For this review, take the finished solid that the model builds, in its own axes (mm). Face numbers are marked on the shaded views. Coordinates: 2 decimals unless noted, no trailing zeros. Order: outer loops, then holes, each group sorted by start corner. A loop starts at its lowest first (then second) coordinate and runs counter-clockwise, first axis right, second up. Notation, with made-up numbers: M -24,-33 L 8,-33 A20 cw 8,-29 Z; hole C 86,-33.75 d10. An arc over 180 degrees is marked long. Use one line per item in the form item = value. Start each with the question number.
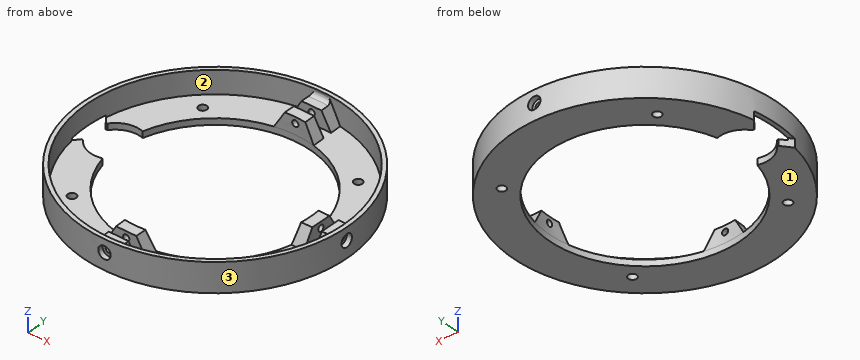
```python
from build123d import *
from OCP.BRepFilletAPI import BRepFilletAPI_MakeChamfer

# Parameters (mm, degrees)
CUT_EXTRUDE1_DEPTH             = 4
CHAMFER1_SIZE                  = 4.528404541
BOSS_EXTRUDE1_START            = 8
BOSS_EXTRUDE1_DEPTH            = 8
CHAMFER2_SIZE                  = 8
CHAMFER2_SIZE_2                = 4.618802154
CIRPATTERN1_COUNT              = 3
CIRPATTERN1_ANGLE              = 180
CHAMFER2_OF_CIRPATTERN1_SIZE   = 8
CHAMFER2_OF_CIRPATTERN1_SIZE_2 = 4.618802154
FILLET1_R                      = 2
SKETCH4_R                      = 2
CUT_EXTRUDE2_DEPTH             = 10
SKETCH5_R                      = 1.5
CUT_EXTRUDE3_DEPTH             = 158
SKETCH7_R                      = 3
CUT_EXTRUDE5_DEPTH             = 4
CIRPATTERN3_COUNT              = 3
CIRPATTERN3_ANGLE              = 180


# Some blends are built 0.0001 mm under size
with BuildPart() as part:
    # Sketch1 → Revolve1 (revolve)
    with BuildSketch(Plane(origin=(0, 0, 0), x_dir=(1, 0, 0), z_dir=(0, 1, 0))):
        Polygon((-46, 0), (-46, -3), (-61.5, -3), (-61.5, -14), (-63.5, -14), (-63.5, 0), align=None)
    revolve(axis=Axis((0, 0, 0.5), (0, 0, 1)))

    # Sketch2 → Cut-Extrude1 (cut)
    with BuildSketch(Plane(origin=(0, 0, 0), x_dir=(-1, 0, 0), z_dir=(0, 0, -1))):
        with BuildLine():
            Line((57.746794345, 7), (73.255615774, 7))
            Line((73.255615774, 7), (73.255615774, -7))
            Line((73.255615774, -7), (57.746794345, -7))
            ThreePointArc((57.746794345, -7), (36, 0), (57.746794345, 7))
        make_face()
    extrude(amount=-CUT_EXTRUDE1_DEPTH, mode=Mode.SUBTRACT)

    # Chamfer1
    # the kernel refuses this chamfer: 5, 4.528404541 mm, written as the material it takes off along each edge
    with BuildSketch(Plane(origin=(-63.112993908, -7, 4), x_dir=(1, 0, 0), z_dir=(0, 0, -1))) as chamfer1_piece_1:
        with BuildLine():
            Line((CHAMFER1_SIZE, 0), (0.712866483, 4.767501749))
            ThreePointArc((0.712866483, 4.767501749), (0.321261242, 2.457711608), (0, 0))
            Line((0, 0), (CHAMFER1_SIZE, 0))
        make_face()
    extrude(amount=16.39656237, mode=Mode.SUBTRACT)
    with BuildSketch(Plane(origin=(-63.112993908, 7, 4), x_dir=(1, 0, 0), z_dir=(0, 0, -1))) as chamfer1_piece_2:
        with BuildLine():
            Line((CHAMFER1_SIZE, 0), (0.712866483, -4.767501749))
            ThreePointArc((0.712866483, -4.767501749), (0.321261242, -2.457711608), (0, 0))
            Line((0, 0), (CHAMFER1_SIZE, 0))
        make_face()
    extrude(amount=16.39656237, mode=Mode.SUBTRACT)

    # Sketch3 → Boss-Extrude1 (add)
    with BuildSketch(Plane.XY.offset(3).offset(BOSS_EXTRUDE1_START)):
        with BuildLine():
            Line((-9.502273243, -50.959479433), (-9.711670224, -44.963134471))
            ThreePointArc((-9.711670224, -44.963134471), (-0.109415415, -45.999869872), (9.497662676, -45.008825842))
            Line((9.497662676, -45.008825842), (9.497662676, -51.008825842))
            Line((9.497662676, -51.008825842), (-9.502273243, -50.959479433))
        make_face()
        with BuildLine():
            Line((9.497662676, -55.408840682), (-9.348607402, -55.359893372))
            Line((-9.348607402, -55.359893372), (-9.158135478, -60.814295643))
            ThreePointArc((-9.158135478, -60.814295643), (0.171750649, -61.499760176), (9.497662676, -60.762195514))
            Line((9.497662676, -60.762195514), (9.497662676, -55.408840682))
        make_face()
    boss_extrude1 = extrude(amount=-BOSS_EXTRUDE1_DEPTH)

    # Chamfer2
    chamfer2_edges_1 = [part.edges().sort_by_distance(p)[0] for p in [
        (-9.25337144, -58.087094508, 11),
    ]]
    chamfer2_side_1 = [part.faces().sort_by_distance(p)[0] for p in [
        (-9.25337144, -58.087094508, 10.907623957),
    ]]
    chamfer2_edges_2 = [part.edges().sort_by_distance(p)[0] for p in [
        (-9.606971733, -47.961306952, 11),
    ]]
    chamfer2_side_2 = [part.faces().sort_by_distance(p)[0] for p in [
        (-9.606971733, -47.961306952, 10.907623957),
    ]]
    chamfer2_edges_3 = [part.edges().sort_by_distance(p)[0] for p in [
        (9.497662676, -48.008825842, 11),
    ]]
    chamfer2_side_3 = [part.faces().sort_by_distance(p)[0] for p in [
        (9.497662676, -48.008825842, 10.907623957),
    ]]
    chamfer2_edges_4 = [part.edges().sort_by_distance(p)[0] for p in [
        (9.497662676, -58.085518098, 11),
    ]]
    chamfer2_side_4 = [part.faces().sort_by_distance(p)[0] for p in [
        (9.497662676, -58.085518098, 10.907623957),
    ]]
    chamfer2 = BRepFilletAPI_MakeChamfer(part.part.solid().wrapped)
    for e in chamfer2_edges_1:
        chamfer2.Add(CHAMFER2_SIZE - 0.0001, CHAMFER2_SIZE_2 - 0.0001, e.wrapped, chamfer2_side_1[0].wrapped)
    for e in chamfer2_edges_2:
        chamfer2.Add(CHAMFER2_SIZE - 0.0001, CHAMFER2_SIZE_2 - 0.0001, e.wrapped, chamfer2_side_2[0].wrapped)
    for e in chamfer2_edges_3:
        chamfer2.Add(CHAMFER2_SIZE - 0.0001, CHAMFER2_SIZE_2 - 0.0001, e.wrapped, chamfer2_side_3[0].wrapped)
    for e in chamfer2_edges_4:
        chamfer2.Add(CHAMFER2_SIZE - 0.0001, CHAMFER2_SIZE_2 - 0.0001, e.wrapped, chamfer2_side_4[0].wrapped)
    add(Compound.cast(chamfer2.Shape()), mode=Mode.REPLACE)  # a hair under: the kernel refuses the full size

    # CirPattern1: Boss-Extrude1 ×3 about axis
    cirpattern1_axis = Axis((0, 0, 0), (0, 0, 1))
    for i in range(1, CIRPATTERN1_COUNT):
        add(boss_extrude1.rotate(cirpattern1_axis, i * CIRPATTERN1_ANGLE / (CIRPATTERN1_COUNT - 1)))

    # Chamfer2 of CirPattern1
    chamfer2_of_cirpattern1_edges_1 = [part.edges().sort_by_distance(p)[0] for p in [
        (58.087094508, -9.25337144, 11),
    ]]
    chamfer2_of_cirpattern1_side_1 = [part.faces().sort_by_distance(p)[0] for p in [
        (58.087094508, -9.25337144, 10.907623957),
    ]]
    chamfer2_of_cirpattern1_edges_2 = [part.edges().sort_by_distance(p)[0] for p in [
        (47.961306952, -9.606971733, 11),
    ]]
    chamfer2_of_cirpattern1_side_2 = [part.faces().sort_by_distance(p)[0] for p in [
        (47.958083075, -9.514651963, 11),
    ]]
    chamfer2_of_cirpattern1_edges_3 = [part.edges().sort_by_distance(p)[0] for p in [
        (48.008825842, 9.497662676, 11),
    ]]
    chamfer2_of_cirpattern1_side_3 = [part.faces().sort_by_distance(p)[0] for p in [
        (48.008825842, 9.497662676, 10.907623957),
    ]]
    chamfer2_of_cirpattern1_edges_4 = [part.edges().sort_by_distance(p)[0] for p in [
        (58.085518098, 9.497662676, 11),
    ]]
    chamfer2_of_cirpattern1_side_4 = [part.faces().sort_by_distance(p)[0] for p in [
        (58.085518098, 9.497662676, 10.907623957),
    ]]
    chamfer2_of_cirpattern1_edges_5 = [part.edges().sort_by_distance(p)[0] for p in [
        (9.25337144, 58.087094508, 11),
    ]]
    chamfer2_of_cirpattern1_side_5 = [part.faces().sort_by_distance(p)[0] for p in [
        (9.25337144, 58.087094508, 10.907623957),
    ]]
    chamfer2_of_cirpattern1_edges_6 = [part.edges().sort_by_distance(p)[0] for p in [
        (9.606971733, 47.961306952, 11),
    ]]
    chamfer2_of_cirpattern1_side_6 = [part.faces().sort_by_distance(p)[0] for p in [
        (9.606971733, 47.961306952, 10.907623957),
    ]]
    chamfer2_of_cirpattern1_edges_7 = [part.edges().sort_by_distance(p)[0] for p in [
        (-9.497662676, 48.008825842, 11),
    ]]
    chamfer2_of_cirpattern1_side_7 = [part.faces().sort_by_distance(p)[0] for p in [
        (-9.497662676, 48.008825842, 10.907623957),
    ]]
    chamfer2_of_cirpattern1_edges_8 = [part.edges().sort_by_distance(p)[0] for p in [
        (-9.497662676, 58.085518098, 11),
    ]]
    chamfer2_of_cirpattern1_side_8 = [part.faces().sort_by_distance(p)[0] for p in [
        (-9.497662676, 58.085518098, 10.907623957),
    ]]
    chamfer2_of_cirpattern1 = BRepFilletAPI_MakeChamfer(part.part.solid().wrapped)
    for e in chamfer2_of_cirpattern1_edges_1:
        chamfer2_of_cirpattern1.Add(CHAMFER2_OF_CIRPATTERN1_SIZE - 0.0001, CHAMFER2_OF_CIRPATTERN1_SIZE_2 - 0.0001, e.wrapped, chamfer2_of_cirpattern1_side_1[0].wrapped)
    for e in chamfer2_of_cirpattern1_edges_2:
        chamfer2_of_cirpattern1.Add(CHAMFER2_OF_CIRPATTERN1_SIZE_2 - 0.0001, CHAMFER2_OF_CIRPATTERN1_SIZE - 0.0001, e.wrapped, chamfer2_of_cirpattern1_side_2[0].wrapped)
    for e in chamfer2_of_cirpattern1_edges_3:
        chamfer2_of_cirpattern1.Add(CHAMFER2_OF_CIRPATTERN1_SIZE - 0.0001, CHAMFER2_OF_CIRPATTERN1_SIZE_2 - 0.0001, e.wrapped, chamfer2_of_cirpattern1_side_3[0].wrapped)
    for e in chamfer2_of_cirpattern1_edges_4:
        chamfer2_of_cirpattern1.Add(CHAMFER2_OF_CIRPATTERN1_SIZE - 0.0001, CHAMFER2_OF_CIRPATTERN1_SIZE_2 - 0.0001, e.wrapped, chamfer2_of_cirpattern1_side_4[0].wrapped)
    for e in chamfer2_of_cirpattern1_edges_5:
        chamfer2_of_cirpattern1.Add(CHAMFER2_OF_CIRPATTERN1_SIZE - 0.0001, CHAMFER2_OF_CIRPATTERN1_SIZE_2 - 0.0001, e.wrapped, chamfer2_of_cirpattern1_side_5[0].wrapped)
    for e in chamfer2_of_cirpattern1_edges_6:
        chamfer2_of_cirpattern1.Add(CHAMFER2_OF_CIRPATTERN1_SIZE - 0.0001, CHAMFER2_OF_CIRPATTERN1_SIZE_2 - 0.0001, e.wrapped, chamfer2_of_cirpattern1_side_6[0].wrapped)
    for e in chamfer2_of_cirpattern1_edges_7:
        chamfer2_of_cirpattern1.Add(CHAMFER2_OF_CIRPATTERN1_SIZE - 0.0001, CHAMFER2_OF_CIRPATTERN1_SIZE_2 - 0.0001, e.wrapped, chamfer2_of_cirpattern1_side_7[0].wrapped)
    for e in chamfer2_of_cirpattern1_edges_8:
        chamfer2_of_cirpattern1.Add(CHAMFER2_OF_CIRPATTERN1_SIZE - 0.0001, CHAMFER2_OF_CIRPATTERN1_SIZE_2 - 0.0001, e.wrapped, chamfer2_of_cirpattern1_side_8[0].wrapped)
    add(Compound.cast(chamfer2_of_cirpattern1.Shape()), mode=Mode.REPLACE)  # a hair under: the kernel refuses the full size

    # Fillet1
    fillet1_edges = [part.edges().sort_by_distance(p)[0] for p in [
        (0.180770138, -61.499734326, 11),
        (61.499734326, 0.180770138, 11),
        (-0.180770138, 61.499734326, 11),
    ]]
    fillet(fillet1_edges, radius=FILLET1_R)

    # Sketch4 → Cut-Extrude2 (cut)
    with BuildSketch(Plane(origin=(0, 0, 0), x_dir=(-1, 0, 0), z_dir=(0, 0, -1))):
        with Locations((-37.476659403, 37.476659403)):
            Circle(SKETCH4_R)
        with Locations((37.476659403, 37.476659403)):
            Circle(SKETCH4_R)
        with Locations((37.476659403, -37.476659403)):
            Circle(SKETCH4_R)
        with Locations((-37.476659403, -37.476659403)):
            Circle(SKETCH4_R)
    extrude(amount=-CUT_EXTRUDE2_DEPTH, mode=Mode.SUBTRACT)

    # Sketch5 → Cut-Extrude3 (cut)
    with BuildSketch(Plane(origin=(0, 0, 0), x_dir=(1, 0, 0), z_dir=(0, 1, 0))):
        with Locations(Location((0, -8, 0), (0, 0, 270))):
            Circle(SKETCH5_R)
    cut_extrude3 = extrude(amount=-CUT_EXTRUDE3_DEPTH, mode=Mode.SUBTRACT)

    # Sketch7 → Cut-Extrude5 (cut)
    with BuildSketch(Plane(origin=(0, -65, 0), x_dir=(1, 0, 0), z_dir=(0, 1, 0))):
        with Locations(Location((0, -8, 0), (0, 0, 90))):
            Circle(SKETCH7_R)
    cut_extrude5 = extrude(amount=CUT_EXTRUDE5_DEPTH, mode=Mode.SUBTRACT)

    # CirPattern3: Cut-Extrude3, Cut-Extrude5 ×3 about axis
    cirpattern3_axis = Axis((0, 0, 0), (0, 0, 1))
    add([cut_extrude3.rotate(cirpattern3_axis, i * CIRPATTERN3_ANGLE / (CIRPATTERN3_COUNT - 1)) for i in range(1, CIRPATTERN3_COUNT)], mode=Mode.SUBTRACT)
    add([cut_extrude5.rotate(cirpattern3_axis, i * CIRPATTERN3_ANGLE / (CIRPATTERN3_COUNT - 1)) for i in range(1, CIRPATTERN3_COUNT)], mode=Mode.SUBTRACT)


solid = part.part
```
1. The part is to be moulded in two halves that separate along X. For the marked faces 1, 2 and 3, say which applies: pulls with the +X half, pulls with the -X half, needs draft (parallel to the pull), parting line crosses it, or undercut.
2. To check wall thickness, follow line 1 (Z direction, x = 58, y = 0); line 2 (X direction, y = 48, z = 8); line 3 (Y direction, x = 26, z = 1.5). State the ranges of each line that lie inside material, in increasing order.
3. Consider section A-A, the plane x = -7. Write out the cut boundary in (y, z).
4. Consider section B-B, the plane y = 0. Write out the cut boundary in (x, z).
5. For pin 1 Ø10 at (x, y) = (42, 36) entering from +Z; pin 2 Ø2 at (y, z) = (-46, 1.5) entering from +X; pin 3 Ø1.8 at (x, z) = (-1, 7.5) entering from +Y, all flat-tipped, find the tip position at first contact; note any pin that passes through.
6. Consider section D-D, the plane y = 43. Write out the cut boundary in (x, z).
Answers follow:
q1.face_1 = needs draft
q1.face_2 = undercut
q1.face_3 = parting line crosses it
q2.line_1 = 0 to 6.5, 9.5 to 11
q2.line_2 = -41.57 to -38.45, -6.61 to -1.5, 1.5 to 6.72, 38.45 to 41.57
q2.line_3 = -57.93 to -37.95, 37.95 to 57.93
q3.outline = M -63.11,0 L -45.46,0 L -45.46,7.66 L -50.97,7.33 L -50.97,3 L -55.37,3 L -55.37,7.07 L -61.1,6.72 L -61.1,14 L -63.11,14 Z; M 45.46,0 L 63.11,0 L 63.11,14 L 61.1,14 L 61.1,7.33 L 55.4,7.33 L 55.4,3 L 51,3 L 51,7.33 L 45.46,7.33 Z
q4.outline = M -63.5,4 L -61.5,4 L -61.5,14 L -63.5,14 Z; M 46,0 L 63.5,0 L 63.5,5 L 61,5 L 61,6.5 L 55.38,6.5 L 55.38,3 L 50.98,3 L 50.98,6.5 L 46,6.5 Z; M 46,9.5 L 50.98,9.5 L 50.98,11 L 46,11 Z; M 55.38,9.5 L 61,9.5 L 61,11 L 63.5,11 L 63.5,14 L 61.5,14 L 61.5,13 A2 cw 59.5,11 L 55.38,11 Z
q5.pin_1 = 3
q5.pin_2 = 44.8
q5.pin_3 = 61
q6.outline = M -46.73,0 L -16.34,0 L -16.34,3 L -43.97,3 L -43.97,14 L -46.73,14 Z; M 16.34,0 L 46.73,0 L 46.73,14 L 43.97,14 L 43.97,3 L 16.34,3 Z
